```python
from build123d import *

# Parameters (mm, degrees)
SKETCH2_W           = 114.3
SKETCH2_H           = 114.3
BOSS_EXTRUDE1_DEPTH = 6.35
SKETCH3_R           = 3.175
CUT_EXTRUDE1_DEPTH  = 7.35
SKETCH3_3_R         = 3.175
CUT_EXTRUDE2_DEPTH  = 7.35
SKETCH3_4_R         = 3.175
CUT_EXTRUDE3_DEPTH  = 7.35
SKETCH3_5_W         = 12.7
SKETCH3_5_H         = 25.4
CUT_EXTRUDE4_DEPTH  = 7.35
SKETCH3_6_W         = 12.7
SKETCH3_6_H         = 25.4
CUT_EXTRUDE5_DEPTH  = 7.35
SKETCH3_7_R         = 3.175
CUT_EXTRUDE6_DEPTH  = 7.35
SHELL1_T            = -2.54
FILLET1_R           = 5


with BuildPart() as part:
    # Sketch2 → Boss-Extrude1 (new body)
    with BuildSketch(Plane.XY):
        with Locations((57.15, 57.15)):
            Rectangle(SKETCH2_W, SKETCH2_H)
    extrude(amount=BOSS_EXTRUDE1_DEPTH)

    # Sketch3 → Cut-Extrude1 (cut, through all)
    with BuildSketch(Plane.XY.offset(6.35)):
        with Locations((31.75, 88.9)):
            Circle(SKETCH3_R)
    extrude(amount=-CUT_EXTRUDE1_DEPTH, mode=Mode.SUBTRACT)

    # Sketch3_3 → Cut-Extrude2 (cut, through all)
    with BuildSketch(Plane.XY.offset(6.35)):
        with Locations((82.55, 88.9)):
            Circle(SKETCH3_3_R)
    extrude(amount=-CUT_EXTRUDE2_DEPTH, mode=Mode.SUBTRACT)

    # Sketch3_4 → Cut-Extrude3 (cut, through all)
    with BuildSketch(Plane.XY.offset(6.35)):
        with Locations((31.75, 25.4)):
            Circle(SKETCH3_4_R)
    extrude(amount=-CUT_EXTRUDE3_DEPTH, mode=Mode.SUBTRACT)

    # Sketch3_5 → Cut-Extrude4 (cut, through all)
    with BuildSketch(Plane.XY.offset(6.35)):
        with Locations((31.75, 57.15)):
            Rectangle(SKETCH3_5_W, SKETCH3_5_H)
    extrude(amount=-CUT_EXTRUDE4_DEPTH, mode=Mode.SUBTRACT)

    # Sketch3_6 → Cut-Extrude5 (cut, through all)
    with BuildSketch(Plane.XY.offset(6.35)):
        with Locations((82.55, 57.15)):
            Rectangle(SKETCH3_6_W, SKETCH3_6_H)
    extrude(amount=-CUT_EXTRUDE5_DEPTH, mode=Mode.SUBTRACT)

    # Sketch3_7 → Cut-Extrude6 (cut, through all)
    with BuildSketch(Plane.XY.offset(6.35)):
        with Locations((82.55, 25.4)):
            Circle(SKETCH3_7_R)
    extrude(amount=-CUT_EXTRUDE6_DEPTH, mode=Mode.SUBTRACT)

    # Shell1
    shell1_openings = [part.faces().sort_by_distance(p)[0] for p in [
        (85.725, 25.4, 6.35),
    ]]
    offset(amount=SHELL1_T, openings=shell1_openings, kind=Kind.INTERSECTION)

    # Fillet1
    fillet1_edges = [part.edges().sort_by_distance(p)[0] for p in [
        (57.15, 114.3, 0),
        (114.3, 57.15, 0),
        (57.15, 0, 0),
        (0, 57.15, 0),
    ]]
    fillet(fillet1_edges, radius=FILLET1_R)


solid = part.part
```
Read the model definition and answer for the solid it produces. Units are mm, in the model's axes. A direction names the side the tool comes from. Coordinates: 2 decimals unless noted, no trailing zeros. Loops run counter-clockwise (first coordinate to the right, second up) from the corner with the lowest first, then second, coordinate; pieces in that order, holes last.
(1) A tool of negligible diameter and unlimited length cuts with its end or side. For faces 5 (the face through (85, 23, 6.35)), 6 (the face through (25.4, 57, 3)), 7 (the face through (32, 72.39, 4)), from which of +Z, -Z, +X, -X, +Y, -Y can it reach the whole face along a straight path? Write none if from no direction.
Solution:
face 5: +Z, +X, -X, +Y, -Y
face 6: +Z, -Z
face 7: +Z
(2) The part is cut by section D-D (x = 54). Determine the outline of the cut face in (y, z), and give its area (3 significant figures).
Solution:
outline: (0, 5) arc R5 ccw to (5, 0) - (109.3, 0) arc R5 ccw to (114.3, 5) - (114.3, 6.35) - (111.76, 6.35) - (111.76, 2.54) - (2.54, 2.54) - (2.54, 6.35) - (0, 6.35) - close
area: 299 mm2
(3) The part is cut by section A-A (z = 3.5). Count the separate pieces of the cut face and the enclosed holes in it, and give its area (3 significant figures).
Solution:
separate pieces: 7
enclosed holes: 7
area: 1,750 mm2
(4) Flat-ended cylindrical pins translate along their axes: pin 1 Ø1 at (y, z) = (63.5, 2.5) entering from -X; pin 2 Ø3 at (y, z) = (67.5, 0.5) entering from +X; pin 3 Ø3 at (x, y) = (48, 53) entering from +Z. Find the tip coordinate at first contact, or state that the pin passes through.
Solution:
pin 1: stops at x = 0.42
pin 2: stops at x = 113.3
pin 3: stops at z = 2.54
(5) The mould has two halves that part along X. Classify faces 1 (the face through (1, 58, 2)), 2 (the face through (34.2, 22.9, 6.35)), 3 (the face through (56, 58, 2.54)), 4 (the face through (32, 41.91, 4)): released by +X, released by -X, zero draft, split by the parting line, or undercut.
Solution:
face 1: released by -X
face 2: zero draft
face 3: undercut
face 4: undercut
(6) The part is cut by section B-B (y = 25.4). Determine the outline of the cut face in (x, z) (3 decimals), and give its area (3 significant figures).
Solution:
outline: (0, 5) arc R5 ccw to (5, 0) - (28.575, 0) - (28.575, 6.35) - (26.035, 6.35) - (26.035, 2.54) - (2.54, 2.54) - (2.54, 6.35) - (0, 6.35) - close; (34.925, 0) - (79.375, 0) - (79.375, 6.35) - (76.835, 6.35) - (76.835, 2.54) - (37.465, 2.54) - (37.465, 6.35) - (34.925, 6.35) - close; (85.725, 0) - (109.3, 0) arc R5 ccw to (114.3, 5) - (114.3, 6.35) - (111.76, 6.35) - (111.76, 2.54) - (88.265, 2.54) - (88.265, 6.35) - (85.725, 6.35) - close
area: 305 mm2
(7) Consider line 1 along X through (y, z) = (65.5, 5); line 2 along X through (y, z) = (25.5, 5); line 3 along Y through (x, z) = (61, 6). Determine where each line is inside the solid, lowest interval first.
Solution:
line 1: x = 0 to 2.54, 22.86 to 25.4, 38.1 to 40.64, 73.66 to 76.2, 88.9 to 91.44, 111.76 to 114.3
line 2: x = 0 to 2.54, 26.04 to 28.58, 34.92 to 37.46, 76.84 to 79.38, 85.72 to 88.26, 111.76 to 114.3
line 3: y = 0 to 2.54, 111.76 to 114.3
